```python
from build123d import *

# Parameters (mm, degrees)
ESQUISSE1_W             = 35.4
ESQUISSE1_H             = 35.4
BOSS_EXTRU_1_DEPTH      = 4
CONG_1_R                = 2
ESQUISSE2_R             = 1.75
ENL_V_MAT_EXTRU_1_DEPTH = 2


with BuildPart() as part:
    # Esquisse1 → Boss.-Extru.1 (new body)
    with BuildSketch(Plane(origin=(0, 0, 0), x_dir=(1, 0, 0), z_dir=(0, 1, 0))):
        Rectangle(ESQUISSE1_W, ESQUISSE1_H)
    extrude(amount=BOSS_EXTRU_1_DEPTH)

    # Congé1
    cong_1_edges = [part.edges().sort_by_distance(p)[0] for p in [
        (0, 0, 17.7),
        (-17.7, 0, 0),
        (0, 0, -17.7),
        (17.7, 0, 0),
        (17.7, 2, 17.7),
        (-17.7, 2, 17.7),
        (-17.7, 2, -17.7),
        (17.7, 2, -17.7),
    ]]
    fillet(cong_1_edges, radius=CONG_1_R)

    # Esquisse2 → Enlèv. mat.-Extru.1 (cut)
    with BuildSketch(Plane(origin=(0, 4, 0), x_dir=(1, 0, 0), z_dir=(0, 1, 0))):
        with Locations(Location((-15.5, 15.5, 0), (0, 0, 270))):
            Circle(ESQUISSE2_R)
        with Locations(Location((15.5, 15.5, 0), (0, 0, 270))):
            Circle(ESQUISSE2_R)
        with Locations(Location((15.5, -15.5, 0), (0, 0, 270))):
            Circle(ESQUISSE2_R)
        with Locations(Location((-15.5, -15.5, 0), (0, 0, 270))):
            Circle(ESQUISSE2_R)
    extrude(amount=-ENL_V_MAT_EXTRU_1_DEPTH, mode=Mode.SUBTRACT)


solid = part.part
```
Can you work these out from the model? Positions are in its coordinate system, mm. A direction names the side the tool comes from. Coordinates: 2 decimals unless noted, no trailing zeros. Write each loop counter-clockwise with the first axis right and the second up, starting at its lowest first coordinate (ties: lowest second). Pieces come first, ordered by that corner, then holes. Notation, with made-up numbers: M -13,81.25 L 44,81.25 A13 cw 44,87.25 Z; hole C -22.75,29.25 d3. An arc over 180 degrees is marked long. Write item = value, one per line. Start each with the question number.
Q1. If we section it at B-B, the plane z = 15: Write out the boundary of the cut face in (x, y).
Q2. If we section it at A-A, the plane y = 2.8: Write out the boundary of the cut face in (x, z), then the cut area to 3 significant figures.
Q3. If we section it at C-C, the plane y = 0.5: Write out the boundary of the cut face in (x, z), then the cut area to 3 significant figures.
Q4. Thinking about a two-plate mould opening in Z: for faces 3 (the face through (0, 0, 0)), 4 (the face through (-13.765, 3.014, 15.272)), 5 (the face through (17.1, 3.01, 17.13)), which applies, released by +Z, released by -Z, zero draft, split by the parting line, or undercut?
Q5. If I drill on L1, parallel to X at y = 3.4, z = 15.5; L2, parallel to Z at x = 15, y = 3.85; L3, parallel to Z at x = 10.5, y = 1.85, over which ranges is the centre line in solid material (lowest first)? Write a range as [from, to].
Q6. I'm going to push flat-ended pins straight in: pin 1 (3 mm diameter, centred on x = -15.5, z = -15.5, fed in from +Y); pin 2 (1 mm diameter, centred on y = 0.5, z = 5.5, fed in from +X); pin 3 (1 mm diameter, centred on x = -9.5, y = 1, fed in from -Z). Where does each tip first touch, or does it pass through?
Q7. On a 3-axis mill with a long thin cutter (end or side, diameter ignored), from which of +Z, -Z, +X, -X, +Y, -Y can I reach the whole of each face in a straight line? I mean faces 1 (the face through (-17.13, 0.6, -0.22)), 2 (the face through (17.235, 3.014, 15.272)). Say none if no direction works.
Check sheet entries:
q1.outline = M -17.7,2 A2 ccw -15.7,0 L 15.7,0 A2 ccw 17.7,2 L 17.7,4 L 17.18,4 L 17.18,2 L 13.82,2 L 13.82,4 L -13.82,4 L -13.82,2 L -17.18,2 L -17.18,4 L -17.7,4 Z
q2.outline = M -17.7,-15.7 A2 ccw -15.7,-17.7 L 15.7,-17.7 A2 ccw 17.7,-15.7 L 17.7,15.7 A2 ccw 15.7,17.7 L -15.7,17.7 A2 ccw -17.7,15.7 Z; hole C -15.5,-15.5 d3.5; hole C -15.5,15.5 d3.5; hole C 15.5,-15.5 d3.5; hole C 15.5,15.5 d3.5
q2.area = 1,210 mm²
q3.outline = M -17.02,-15.7 A1.32 ccw -15.7,-17.02 L 15.7,-17.02 A1.32 ccw 17.02,-15.7 L 17.02,15.7 A1.32 ccw 15.7,17.02 L -15.7,17.02 A1.32 ccw -17.02,15.7 Z
q3.area = 1,160 mm²
q4.face_3 = zero draft
q4.face_4 = undercut
q4.face_5 = released by +Z
q5.L1 = [-17.7, -17.25], [-13.75, 13.75], [17.25, 17.7]
q5.L2 = [-17.7, -17.18], [-13.82, 13.82], [17.18, 17.7]
q5.L3 = [-17.69, 17.69]
q6.pin_1 = 2
q6.pin_2 = 17.43
q6.pin_3 = -17.64
q7.face_1 = +Z, -Z, -X, -Y
q7.face_2 = +Y
